Build history of the part. All positions in model axes, mm. Round coordinates to 2 decimals unless told otherwise and drop trailing zeros. Write each loop counter-clockwise with the first axis right and the second up, starting at its lowest first coordinate (ties: lowest second). Pieces come first, ordered by that corner, then holes. Notation, with made-up numbers: (67.25, -5) - (98.25, -5) arc R12 ccw to (98.25, 17) - close; hole circle Ø9 at (-34, 27). An arc over 180 degrees is marked (long way). Write each question's results on one line, items separated by ' | '.
from build123d import *
from OCP.BRepFilletAPI import BRepFilletAPI_MakeChamfer

# Parameters (mm, degrees)
CHAMFER1_SIZE  = 0.5
CHAMFER2_SIZE  = 0.3
CHAMFER2_SIZE2 = 0.173205081


with BuildPart() as part:
    # Sketch1 → Revolve1 (revolve)
    with BuildSketch(Plane(origin=(0, 0, 0), x_dir=(1, 0, 0), z_dir=(0, 1, 0)), mode=Mode.PRIVATE) as revolve1_sk:
        Polygon((-1, 0), (-4, 0), (-4, -100), (-1, -100), (-1, -98), (0, -98), (0, -2), (-1, -2), align=None)
    revolve(revolve1_sk.sketch.rotate(Axis((0, 0, 98), (0, 0, -1)), 180), axis=Axis((0, 0, 98), (0, 0, -1)))

    # Chamfer1
    chamfer1_edges = [part.edges().sort_by_distance(p)[0] for p in [
        (-4, 0, 100),
        (-4, 0, 0),
    ]]
    chamfer(chamfer1_edges, length=CHAMFER1_SIZE)

    # Chamfer2: one chamfer whose edges measure the first distance from different faces: ONE call of the kernel's chamfer builder (chamfer() names one face for all edges)
    chamfer2_edges_1 = [part.edges().sort_by_distance(p)[0] for p in [
        (-1, 0, 2),
    ]]
    chamfer2_side_1 = [part.faces().sort_by_distance(p)[0] for p in [
        (0, 0, 2),
    ]]
    chamfer2_edges_2 = [part.edges().sort_by_distance(p)[0] for p in [
        (-1, 0, 98),
    ]]
    chamfer2_side_2 = [part.faces().sort_by_distance(p)[0] for p in [
        (-1, 0, 99),
    ]]
    chamfer2_edges_3 = [part.edges().sort_by_distance(p)[0] for p in [
        (-1, 0, 100),
    ]]
    chamfer2_side_3 = [part.faces().sort_by_distance(p)[0] for p in [
        (-3.401005051, 0, 100),
    ]]
    chamfer2_edges_4 = [part.edges().sort_by_distance(p)[0] for p in [
        (-1, 0, 0),
    ]]
    chamfer2_side_4 = [part.faces().sort_by_distance(p)[0] for p in [
        (-1, 0, 1),
    ]]
    chamfer2 = BRepFilletAPI_MakeChamfer(part.part.solid().wrapped)
    for e in chamfer2_edges_1:
        chamfer2.Add(CHAMFER2_SIZE, CHAMFER2_SIZE2, e.wrapped, chamfer2_side_1[0].wrapped)  # the first distance lies on this face
    for e in chamfer2_edges_2:
        chamfer2.Add(CHAMFER2_SIZE, CHAMFER2_SIZE2, e.wrapped, chamfer2_side_2[0].wrapped)  # the first distance lies on this face
    for e in chamfer2_edges_3:
        chamfer2.Add(CHAMFER2_SIZE, CHAMFER2_SIZE2, e.wrapped, chamfer2_side_3[0].wrapped)  # the first distance lies on this face
    for e in chamfer2_edges_4:
        chamfer2.Add(CHAMFER2_SIZE, CHAMFER2_SIZE2, e.wrapped, chamfer2_side_4[0].wrapped)  # the first distance lies on this face
    add(Compound.cast(chamfer2.Shape()), mode=Mode.REPLACE)


solid = part.part
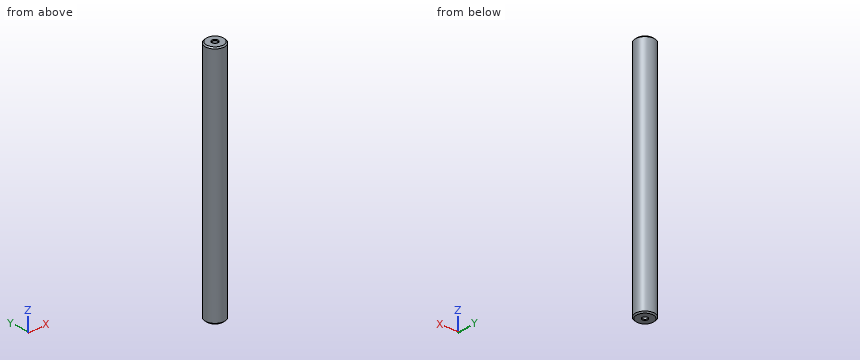
(1) Flat gauge pins, fed straight in: pin 1 Ø1.8 at (x, y) = (0, 0) entering from -Z; pin 2 Ø1.1 at (x, y) = (0, 0) entering from -Z; pin 3 Ø1 at (y, z) = (1.5, 21) entering from -X. Where does each tip first touch, or does it go through?
Worked answers:
pin 1: stops at z = 1.88 | pin 2: stops at z = 2 | pin 3: stops at x = -3.87
(2) Slice it at A-A, the plane z = 20.5. Write the cut outline in (x, y).
Worked answers:
outline: circle Ø8 at (0, 0)
(3) Drill centre lines: probe 1 along Y at (x, z) = (0, 1.4); probe 2 along Z at (x, y) = (-1.25, -0.25); probe 3 along Y at (x, z) = (0.75, 89.5). Where is each one in solid material? Low to high. Write a range as [from, to].
Worked answers:
probe 1: y = [-4, -1], [1, 4] | probe 2: z = [0, 99.99] | probe 3: y = [-3.93, 3.93]
